Solid Edge part; units mm, degrees
sketch "Sketch1" plane through (0, 0, 0) normal (0, -1, 0) x (1, 0, 0)
  line L0 (12.5, 0) -> (25, -25)
  line L1 (-25, -25) -> (25, -25)
  line L2 (-12.5, 0) -> (-25, -25)
  arc A0 (-12.5, 0) -> (12.5, 0) centre (0, 0) cw
extrude "Protrusion1" add sketch "Sketch1" against normal blind 7
sketch "Sketch2" plane through (0, 0, 0) normal (0, -1, 0) x (1, 0, 0)
  circle A0 centre (0, 0) radius 4.15
extrude "Cutout1" cut sketch "Sketch2" against normal through all
sketch "Sketch3" plane through (0, 7, -6.25) normal (0, 1, 0) x (-1, 0, 0)
  line L0 (-22.5, -13.75) -> (22.5, -13.75)
  line L1 (22.5, -13.75) -> (25, -18.75)
  line L2 (25, -18.75) -> (-25, -18.75)
  line L3 (-25, -18.75) -> (-22.5, -13.75)
extrude "ExtrudedProtrusion_2" add sketch "Sketch3" along normal blind 7.5
sketch "Sketch4" plane through (0, 14.5, -22.5) normal (0, 1, 0) x (-1, 0, 0)
  line L0 (-25, -2.5) -> (-12.5, 22.5)
  line L1 (12.5, 22.5) -> (25, -2.5)
  line L2 (25, -2.5) -> (-25, -2.5)
  arc A0 (-12.5, 22.5) -> (12.5, 22.5) centre (0, 22.5) cw
extrude "ExtrudedProtrusion_3" add sketch "Sketch4" along normal blind 7
sketch "Sketch5" plane through (0, 14.5, -22.5) normal (0, 1, 0) x (-1, 0, 0)
  circle A0 centre (0, 22.5) radius 4.15
extrude "Cutout2" cut sketch "Sketch5" along normal through all
sketch "Sketch6" plane through (0, 10, -20) normal (0, 0, 1) x (-1, 0, 0)
  circle A0 centre (-9.9456, -0.75) radius 2.65
  circle A1 centre (10.0544, -0.75) radius 2.65
extrude "Cutout3" cut sketch "Sketch6" against normal through all
properties material "PLA"
Here's how the part is built. I have some questions about the finished solid (model axes, mm). A direction names the side the tool comes from. Coordinates: 2 decimals unless noted, no trailing zeros. Write each loop counter-clockwise with the first axis right and the second up, starting at its lowest first coordinate (ties: lowest second). Pieces come first, ordered by that corner, then holes. Notation, with made-up numbers: (-23, 23) -> (-2, 23) arc R19 ccw to (-2, 37) -> close; hole circle Ø8 at (-34, -24.75). An arc over 180 degrees is marked (long way). Use a Markdown table: item, result. Add a question column.
(1) If we section it at A-A, the plane x = 0: Write out the boundary of the cut face in (y, z), and give its area (3 significant figures).
(2) For faces 5 (the flat face through (0, 14.5, -7)), 6 (the flat face through (-18.66, 5.82, -12.32)), which set-ups out of +Z, -Z, +X, -X, +Y, -Y let a thin tool reach every point of the face, with its end or its side?
(3) We'd pull the mould along Y, two halves only. Please class faces 1 (the flat face through (0, 7, -8)), 2 (the flat face through (0, 11, -20)), 3 (the flat face through (0, 21.5, -10)), 4 (the flat face through (0, 0, -11)): +Y half, -Y half, draft (parallel to the pull), parting line (faces both ways), or undercut.
(4) Please list where these lines run through material, in increasing order: line 1 (Z direction, x = 0, y = 17.75); line 2 (X direction, y = 10.75, z = -21.4); line 3 (Y direction, x = -11, z = -7).
(5) I'm going to push flat-ended pins straight in: P1, Ø9.5, axis at x = 0, z = 0, coming from the -Y side; P2, Ø6, axis at y = 7, z = -18.5, coming from the +X side; P3, Ø1.5, axis at y = 5, z = -15, coming from the -X side (3 decimals); P4, Ø4, axis at y = 3, z = -6, coming from the +X side. Where does each tip first touch, or does it pass through?
(6) If we section it at C-C, the plane z = -16.5: Write out the boundary of the cut face in (x, y).
(7) If we section it at D-D, the plane x = -20.5: Write out the boundary of the cut face in (y, z).
(8) If we section it at B-B, the plane y = 10.75: Write out the boundary of the cut face in (x, z), and give its area (4 significant figures).
Outcome:
| question | item | result |
|---|---|---|
| 1 | outline | (0, -25) -> (21.5, -25) -> (21.5, -4.15) -> (14.5, -4.15) -> (14.5, -20) -> (7, -20) -> (7, -4.15) -> (0, -4.15) -> close; (0, 4.15) -> (7, 4.15) -> (7, 12.5) -> (0, 12.5) -> close; (14.5, 4.15) -> (21.5, 4.15) -> (21.5, 12.5) -> (14.5, 12.5) -> close |
| 1 | area | 446 mm^2 |
| 2 | face 5 | +Z, +X, -X |
| 2 | face 6 | +Z, -X, +Y, -Y |
| 3 | face 1 | undercut |
| 3 | face 2 | undercut |
| 3 | face 3 | +Y half |
| 3 | face 4 | -Y half |
| 4 | line 1 | z = -25 to -4.15, 4.15 to 12.5 |
| 4 | line 2 | x = -23.2 to -12.7, -7.4 to 7.3, 12.6 to 23.2 |
| 4 | line 3 | y = 0 to 7, 14.5 to 21.5 |
| 5 | P1 | stops at y = 0 |
| 5 | P2 | stops at x = 23.25 |
| 5 | P3 | stops at x = -20.375 |
| 5 | P4 | stops at x = 16.5 |
| 6 | outline | (-20.75, 0) -> (20.75, 0) -> (20.75, 7) -> (-20.75, 7) -> close; (-20.75, 14.5) -> (20.75, 14.5) -> (20.75, 21.5) -> (-20.75, 21.5) -> close |
| 7 | outline | (0, -25) -> (21.5, -25) -> (21.5, -16) -> (14.5, -16) -> (14.5, -20) -> (7, -20) -> (7, -16) -> (0, -16) -> close |
| 8 | outline | (-25, -25) -> (-12.7, -25) -> (-12.7, -20) -> (-22.5, -20) -> close; (-7.4, -25) -> (7.3, -25) -> (7.3, -20) -> (-7.4, -20) -> close; (12.6, -25) -> (25, -25) -> (22.5, -20) -> (12.6, -20) -> close |
| 8 | area | 184.5 mm^2 |
